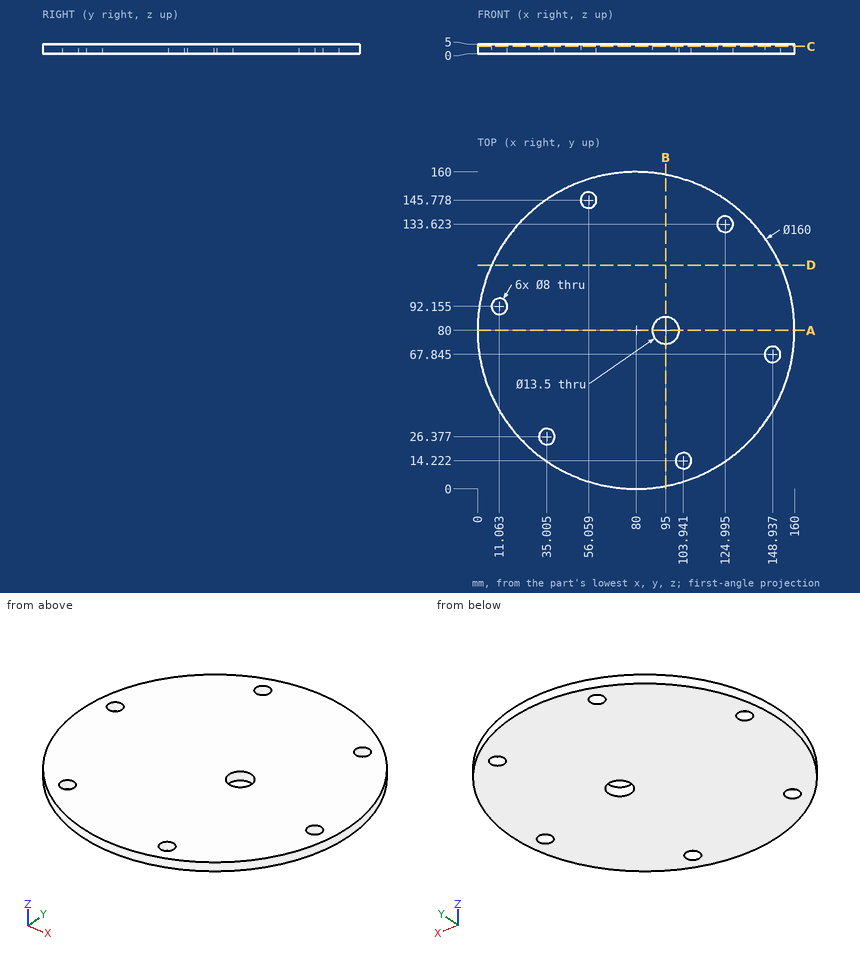
Could you check a few things on this drawing? It's one solid part, dimensions in mm from its lowest x, y, z. Round coordinates to 2 decimals unless told otherwise and drop trailing zeros. Order: outer loops, then holes, each group sorted by start corner. A loop starts at its lowest first (then second) coordinate and runs counter-clockwise, first axis right, second up. Notation, with made-up numbers: M 58.5,9 L 92.5,9 A27 cw 92.5,36 Z; hole C 28.5,33 d9. An arc over 180 degrees is marked long. Use a Markdown table: item, result.
1) I'm going to push flat-ended pins straight in: P1, Ø15.5, axis at x = 95, y = 80, coming from the -Z side; P2, Ø6.5, axis at x = 56.06, y = 145.78, coming from the +Z side; P3, Ø3, axis at x = 63, z = 2.5, coming from the +Y side; P4, Ø1.5, axis at y = 39.5, z = 0.5, coming from the -X side (1 decimal). Where does each tip first touch, or does it pass through?
Geometry says:
| item | result |
|---|---|
| P1 | stops at z = 0 |
| P2 | passes through |
| P3 | stops at y = 158.48 |
| P4 | stops at x = 10.6 |
2) Imagine slicing it at A-A (y = 80). List the corners of the cut face in (x, z) for me.
Geometry says:
| item | result |
|---|---|
| outline | M 0,0 L 88.25,0 L 88.25,5 L 0,5 Z; M 101.75,0 L 160,0 L 160,5 L 101.75,5 Z |
3) If I drill on line 1 along Y through (x, z) = (8.5, 1.2) (1 decimal); line 2 along Y through (x, z) = (79, 3.9); line 3 along Y through (x, z) = (99, 4.7) (1 decimal), over which ranges is the centre line in solid material (lowest first)?
Geometry says:
| item | result |
|---|---|
| line 1 | y = 44.1 to 89.1, 95.2 to 115.9 |
| line 2 | y = 0.01 to 159.99 |
| line 3 | y = 2.3 to 74.6, 85.4 to 157.7 |
4) Imagine slicing it at B-B (x = 95). List the corners of the cut face in (y, z) for me.
Geometry says:
| item | result |
|---|---|
| outline | M 1.42,0 L 73.25,0 L 73.25,5 L 1.42,5 Z; M 86.75,0 L 158.58,0 L 158.58,5 L 86.75,5 Z |
5) Imagine slicing it at D-D (y = 113). List the corners of the cut face in (x, z) for me.
Geometry says:
| item | result |
|---|---|
| outline | M 7.12,0 L 152.88,0 L 152.88,5 L 7.12,5 Z |
6) Imagine slicing it at C-C (z = 3.85). Give the number of separate pieces and of enclosed holes in the cut face, then the cut area to 3 significant figures.
Geometry says:
| item | result |
|---|---|
| separate pieces | 1 |
| enclosed holes | 7 |
| area | 19,700 mm² |
